Work out the finished part from the listing and answer in its coordinate system (mm). Round coordinates to 2 decimals unless told otherwise and drop trailing zeros. Loops run counter-clockwise (first coordinate to the right, second up) from the corner with the lowest first, then second, coordinate; pieces in that order, holes last. Notation, with made-up numbers: M -33,-6.75 L 17,-6.75 A32 cw 17,26.25 Z; hole C -9,-1 d1. An arc over 180 degrees is marked long. One line per item, written item: value.
Autodesk Inventor part; units mm, degrees
ref_plane "YZ Plane" through (0, 0, 0) normal (1, 0, 0) x (0, 1, 0)
ref_plane "XZ Plane" through (0, 0, 0) normal (0, 1, 0) x (-1, 0, 0)
ref_plane "XY Plane" through (0, 0, 0) normal (0, 0, 1) x (1, 0, 0)
sketch "Esquisse1" plane through (0, 0, 0) normal (1, 0, 0) x (0, 1, 0)
  line L0 (0, 0) -> (80, 0)
  line L1 (80, 0) -> (80, -200)
  line L2 (80, -200) -> (0, -200)
  line L3 (0, -200) -> (0, 0)
  dimension "d0" = 80
  dimension "d1" = 200
extrude "Extrusion1" add sketch "Esquisse1" along normal blind 5
sketch "Esquisse3" plane through (5, 0, 0) normal (1, 0, 0) x (0, 0, -1)
  line L0 (0, 0) -> (2.5, 0)
  line L1 (0, 0) -> (200, 0)
  line L2 (2.5, 0) -> (2.5, 40)
  line L3 (100, 0) -> (100, 21.0843)
  point P0 (2.5, 40)
  point P1 (197.5, 40)
  dimension "d15" = 2.5
  dimension "d16" = 40
hole "Perçage2" at (5, 40, -2.5) at (5, 40, -197.5) direction (-1, 0, 0) diameter 2.459 end through all
sketch "Esquisse4" plane through (0, 0, -200) normal (0, -1, 0) x (1, 0, 0)
  line L0 (0, 200) -> (0, 197.5)
  line L1 (0, 0) -> (0, 200)
  line L2 (0, 197.5) -> (2.5, 197.5)
  line L3 (5, 200) -> (5, 0)
  point P0 (2.5, 2.5)
  point P1 (2.5, 100)
  dimension "d24" = 2.5
  dimension "d25" = 2.5
  dimension "d26" = 90
hole "Perçage3" at (2.5, 0, -2.5) at (2.5, 0, -197.5) at (2.5, 0, -100) direction (0, 1, 0) diameter 2.459 depth 8.8 tip angle 118
sketch "Esquisse5" plane through (0, 80, 0) normal (0, 1, 0) x (1, 0, 0)
  line L0 (0, 0) -> (2.5, 0)
  line L1 (0, 0) -> (5, 0)
  line L2 (2.5, 0) -> (2.5, 2.5)
  line L3 (2.5, 0) -> (5, 0) construction
  line L4 (0, 200) -> (0, 0)
  line L5 (0, 100) -> (2.5, 100)
  point P0 (2.5, 197.5)
  dimension "d34" = 2.5
  dimension "d35" = 90
hole "Perçage4" at (2.5, 80, -2.5) at (2.5, 80, -197.5) at (2.5, 80, -100) direction (0, -1, 0) diameter 2.459 depth 8.8 tip angle 118
sketch "Esquisse7" plane through (5, 0, 0) normal (1, 0, 0) x (0, 0, -1)
  line L0 (0, 0) -> (100, 0)
  line L1 (0, 0) -> (200, 0)
  line L2 (100, 0) -> (180, 0) construction
  line L3 (100, 80) -> (100, 10)
  line L4 (100, 80) -> (170, 80) construction
  line L5 (100, 10) -> (90.8075, 10)
  line L6 (100, 10) -> (80, 10)
  line L7 (80, 10) -> (80, 42)
  point P0 (120, 42)
  dimension "d50" = 100
  dimension "d53" = 70
  dimension "d54" = 90
  dimension "d67" = 20
  dimension "d68" = 32
hole "Perçage6" at (5, 42, -120) at (5, 42, -80) direction (-1, 0, 0) diameter 4.134 end through all
sketch "Esquisse8" plane through (5, 0, 0) normal (1, 0, 0) x (0, 0, -1)
  circle A0 centre (80, 42) radius 2.067
  line L0 (80, 42) -> (100, 42)
  point P0 (0, 0)
  dimension "d69" = 20
hole "Perçage7" at (5, 42, -100) direction (-1, 0, 0) diameter 8.5 end through all
properties part number "chassis_côté"
1) Find the intervals of material crossed by probe 1 along Z at (x, y) = (2.5, 76); probe 2 along Z at (x, y) = (1.7, 6); probe 3 along X at (y, z) = (74.25, -100), in increasing order. Write a range as from..to.
Check values:
probe 1: -200..-198.73, -196.27..-101.23, -98.77..-3.73, -1.27..0
probe 2: -200..-198.43, -196.57..-100.93, -99.07..-3.43, -1.57..0
probe 3: 0..1.27, 3.73..5
2) Each of these flat-tipped pins is pushed along its axis until it touches: pin 1 (1.5 mm diameter, centred on x = 2.5, z = -100, fed in from -Y); pin 2 (1.5 mm diameter, centred on x = 2.5, z = -197.5, fed in from +Y); pin 3 (2 mm diameter, centred on x = 2.5, z = -2.5, fed in from +Y). Where does it stop, or does it pass through?
Check values:
pin 1: y = 9.09
pin 2: y = 70.91
pin 3: y = 71.06
3) The mould has two halves that part along Y. Classify faces 1 (the face through (2.5, 0, -101.4)), 2 (the face through (2.465, 41.909, -77.935)), 3 (the face through (2, 41, -200)): +Y half, -Y half, draft (parallel to the pull), parting line (faces both ways), or undercut.
Check values:
face 1: -Y half
face 2: undercut
face 3: draft
4) Find section A-A (z = -80). Give the vertices of the cut face in (x, y).
Check values:
outline: M 0,0 L 5,0 L 5,39.93 L 0,39.93 Z; M 0,44.07 L 5,44.07 L 5,80 L 0,80 Z
